```python
from build123d import *

# Parameters (mm, degrees)
F0_W     = 64.522118
F0_H     = 110.606628
F1_DEPTH = 20
F2_R     = 12.7
F3_W     = 40.194572
F3_H     = 85.488498
F4_DEPTH = 40.548261


with BuildPart() as f1:
    # F0 (on Top) → F1 (new body)
    with BuildSketch(Plane.XY):
        Rectangle(F0_W, F0_H)
    extrude(amount=F1_DEPTH)

    # F2
    f2_edges = [f1.edges().sort_by_distance(p)[0] for p in [
        (-32.261059, 55.303314, 10),
        (-32.261059, -55.303314, 10),
        (32.261059, 55.303314, 10),
        (32.261059, -55.303314, 10),
    ]]
    fillet(f2_edges, radius=F2_R)

    # F3 (on Top) → F4 (join)
    with BuildSketch(Plane.XY):
        Rectangle(F3_W, F3_H)
    extrude(amount=F4_DEPTH)


solid = f1.part
```
For this review, take the finished solid that the model builds, in its own axes (mm). A direction names the side the tool comes from. Round coordinates to 2 decimals unless told otherwise and drop trailing zeros. Write each loop counter-clockwise with the first axis right and the second up, starting at its lowest first coordinate (ties: lowest second). Pieces come first, ordered by that corner, then holes. Notation, with made-up numbers: (-26.5, -1) - (19.5, -1) arc R30 ccw to (19.5, 22) - close; hole circle Ø9 at (11, 70.5). An arc over 180 degrees is marked (long way). Write each question's results on one line, items separated by ' | '.
Item 1: Take a section at B-B on x = -14. State the section outline as (y, z) points, then the cut area to 3 significant figures.
Calculated:
outline: (-55.3, 0) - (55.3, 0) - (55.3, 20) - (42.74, 20) - (42.74, 40.55) - (-42.74, 40.55) - (-42.74, 20) - (-55.3, 20) - close | area: 3,970 mm^2
Item 2: Take a section at C-C on z = 33. State the section outline as (x, y) points.
Calculated:
outline: (-20.1, -42.74) - (20.1, -42.74) - (20.1, 42.74) - (-20.1, 42.74) - close
Item 3: Take a section at D-D on x = -23. State the section outline as (y, z) points.
Calculated:
outline: (-54.83, 0) - (54.83, 0) - (54.83, 20) - (-54.83, 20) - close
Item 4: Take a section at A-A on y = 9. State the section outline as (x, z) points, then the cut area to 3 significant figures.
Calculated:
outline: (-32.26, 0) - (32.26, 0) - (32.26, 20) - (20.1, 20) - (20.1, 40.55) - (-20.1, 40.55) - (-20.1, 20) - (-32.26, 20) - close | area: 2,120 mm^2
Item 5: For faces 1 (the face through (0, -55.303, 10)), 2 (the face through (0, 42.744, 30)), 3 (the face through (-20.097, -1, 30)), 4 (the face through (0, -42.744, 30)), 5 (the face through (20.097, -1, 30)), list the 3-axis set-ups (+Z, -Z, +X, -X, +Y, -Y) from which the entire face can be reached by the end or side of a thin tool; tool diameter is ignored.
Calculated:
face 1: +Z, -Z, +X, -X, -Y | face 2: +Z, +X, -X, +Y | face 3: +Z, -X, +Y, -Y | face 4: +Z, +X, -X, -Y | face 5: +Z, +X, +Y, -Y
Item 6: To check wall thickness, follow line 1 along Y through (x, z) = (14, 34); line 2 along X through (y, z) = (-4.5, 20.5); line 3 along Z through (x, y) = (26.5, 19). State the ranges of each line that lie inside material, in increasing order. Write a range as from..to.
Calculated:
line 1: y = -42.74..42.74 | line 2: x = -20.1..20.1 | line 3: z = 0..20
Item 7: For pin 1 (1 mm diameter, centred on x = -22, z = 30, fed in from +Y); pin 2 (6 mm diameter, centred on y = 1.5, z = 32, fed in from +X); pin 3 (22.5 mm diameter, centred on y = 0.5, z = 34.5, fed in from -X); pin 4 (1 mm diameter, centred on x = -24, z = 4.5, fed in from -Y), all flat-tipped, find the tip position at first contact; note any pin that passes through.
Calculated:
pin 1: passes through | pin 2: stops at x = 20.1 | pin 3: stops at x = -20.1 | pin 4: stops at y = -54.68
